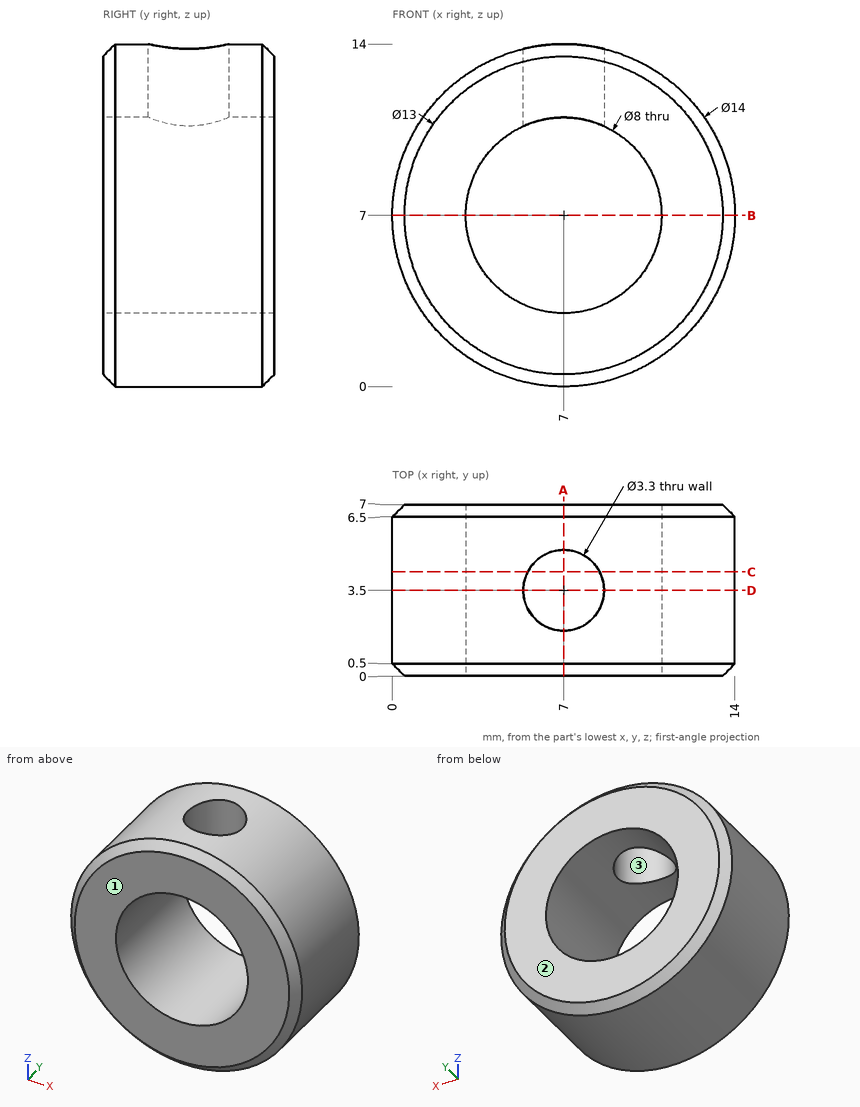
For this review, use the dimensioned drawing (mm, ordinates from the lowest corner) and the shaded views. Round coordinates to 2 decimals unless told otherwise and drop trailing zeros. Write each loop counter-clockwise with the first axis right and the second up, starting at its lowest first coordinate (ties: lowest second). Pieces come first, ordered by that corner, then holes. Notation, with made-up numbers: (-2, 15.5) -> (57, 15.5) arc R32 ccw to (57, 48.5) -> close; hole circle Ø8 at (72, 66.25). An arc over 180 degrees is marked (long way). One line per item, written item: value. Start each with the question number.
Q1. Add section D-D (y = 3.5). Give the boundary of the cut face in (x, z), then the cut area to 3 significant figures.
Q2. Insertion check: P1, Ø1.5, axis at y = 5, z = 5, coming from the +X side; P2, Ø3, axis at x = 7, y = 3.5, coming from the +Z side. Each pin has a flat end and moves straight along its axis. Give the tip position at first contact, or say it passes through.
Q3. Add section B-B (z = 7). Give the boundary of the cut face in (x, y).
Q4. Add section C-C (y = 4.25). Give the boundary of the cut face in (x, z).
Q5. Add section A-A (x = 7). Give the boundary of the cut face in (y, z), then the cut area to 3 significant figures.
Q6. The part is to be moulded in two halves that separate along Y. For the marked faces 1, 2 and 3, say which applies: pulls with the +Y half, pulls with the -Y half, needs draft (parallel to the pull), parting line crosses it, or undercut.
Q7. To check wall thickness, follow probe 1 along X at (y, z) = (2, 7); probe 2 along Z at (x, y) = (8, 5.75); probe 3 along Y at (x, z) = (8, 13). State the ranges of each line that lie inside material, in increasing order.
Response:
1. outline: (5.35, 10.64) -> (5.35, 13.8) arc R7 ccw (long way) to (8.65, 13.8) -> (8.65, 10.64) arc R4 cw (long way) to start
1. area: 93.6 mm^2
2. P1: stops at x = 13.89
2. P2: stops at z = 3.29
3. outline: (0, 0.5) -> (0.5, 0) -> (3, 0) -> (3, 7) -> (0.5, 7) -> (0, 6.5) -> close; (11, 0) -> (13.5, 0) -> (14, 0.5) -> (14, 6.5) -> (13.5, 7) -> (11, 7) -> close
4. outline: (5.53, 10.72) -> (5.53, 13.84) arc R7 ccw (long way) to (8.47, 13.84) -> (8.47, 10.72) arc R4 cw (long way) to start
5. outline: (0, 0.5) -> (0.5, 0) -> (6.5, 0) -> (7, 0.5) -> (7, 3) -> (0, 3) -> close; (0, 11) -> (1.85, 11) -> (1.85, 14) -> (0.5, 14) -> (0, 13.5) -> close; (5.15, 11) -> (7, 11) -> (7, 13.5) -> (6.5, 14) -> (5.15, 14) -> close
5. area: 31.6 mm^2
6. face 1: pulls with the -Y half
6. face 2: pulls with the +Y half
6. face 3: undercut
7. probe 1: x = 0 to 3, 11 to 14
7. probe 2: z = 0.07 to 3.13, 10.87 to 13.93
7. probe 3: y = 0 to 2.19, 4.81 to 7
